Part model, mm, in its own coordinate system. A direction names the side the tool comes from. Round coordinates to 2 decimals unless told otherwise and drop trailing zeros. Write each loop counter-clockwise with the first axis right and the second up, starting at its lowest first coordinate (ties: lowest second). Pieces come first, ordered by that corner, then holes.
Solid Edge part; units mm, degrees
sketch "Sketch1" plane through (0, 0, 0) normal (0, 0, 1) x (1, 0, 0)
  circle A0 centre (0, 0) radius 12.5
  circle A1 centre (0, 0) radius 1.6
extrude "Protrusion1" add sketch "Sketch1" along normal blind 35
sketch "Sketch2" plane through (0, 0, 35) normal (0, 0, 1) x (1, 0, 0)
  circle A0 centre (0, 0) radius 12.5
  circle A1 centre (0, 0) radius 6
extrude "ExtrudedCutout_1" cut sketch "Sketch2" against normal blind 28
sketch "Sketch3" plane through (0, 0, 7) normal (0, 0, 1) x (1, 0, 0)
  circle A0 centre (0, 9.5) radius 1.6
extrude "Cutout1" cut sketch "Sketch3" against normal up to next
sketch "Sketch4" plane through (0, 0, 7) normal (0, 0, 1) x (1, 0, 0)
  circle A0 centre (0, 9.5) radius 3.25
extrude "ExtrudedCutout_3" cut sketch "Sketch4" against normal blind 3.5
pattern_circular "Pattern1" count 4 over 360 about axis through (0, 0, 7) along (0, 0, 1) of "Cutout1", "ExtrudedCutout_3"
hole "Hole_4" at (0, 0, 29) direction (0, 1, 0) diameter 2.013 end up to next
hole "Hole1" at (0, 0, 20) direction (0, 1, 0) diameter 2.013 end up to next
hole "Hole2" at (0, 0, 11) direction (0, 1, 0) diameter 2.013 end up to next
Q1. Cut at B-B on x = 10.5. Write the cut outline in (y, z).
Values follow:
outline: (-6.78, 0) - (-1.25, 0) - (-1.25, 3.5) - (-3.09, 3.5) - (-3.09, 7) - (-6.78, 7) - close; (1.25, 0) - (6.78, 0) - (6.78, 7) - (3.09, 7) - (3.09, 3.5) - (1.25, 3.5) - close
Q2. Cut at A-A on y = 4.5. Write the cut outline in (x, z).
Values follow:
outline: (-11.66, 0) - (11.66, 0) - (11.66, 7) - (3.97, 7) - (3.97, 35) - (-3.97, 35) - (-3.97, 7) - (-11.66, 7) - close; hole circle Ø2.01 at (0, 11); hole circle Ø2.01 at (0, 20); hole circle Ø2.01 at (0, 29)
Q3. Drop flat-ended pins along their axis: pin 1 (12 mm diameter, centred on y = -7, z = 7.5, fed in from +X); pin 2 (4 mm diameter, centred on x = -2.5, y = 10, fed in from +Z); pin 3 (5 mm diameter, centred on y = 2, z = 23, fed in from +X); pin 4 (2.5 mm diameter, centred on x = 9.5, y = 0, fed in from +Z). Give the stop position or say it passes through.
Values follow:
pin 1: stops at x = 12.42
pin 2: stops at z = 7
pin 3: stops at x = 6
pin 4: passes through
Q4. Cut at C-C on y = 9.5. Write the cut outline in (x, z).
Values follow:
outline: (-8.12, 0) - (-1.6, 0) - (-1.6, 3.5) - (-3.25, 3.5) - (-3.25, 7) - (-8.12, 7) - close; (1.6, 0) - (8.12, 0) - (8.12, 7) - (3.25, 7) - (3.25, 3.5) - (1.6, 3.5) - close
Q5. Which spindle directions (+Z, -Z, +X, -X, +Y, -Y) get a long thin tool onto all of the face, cutting with end or side? Do faces 1 (the flat face through (8, -1, 3.5)), 2 (the cylindrical face through (7.94, 0.35, 1.77)), 3 (the cylindrical face through (1, 3.6, 11.1)). Say none if no direction does.
Values follow:
face 1: +Z
face 2: +Z, -Z
face 3: +Y
Q6. Cut at D-D on x = 0. State how many separate pieces and enclosed holes the cut face has, plus the area to 3 significant figures.
Values follow:
separate pieces: 7
enclosed holes: 0
area: 306 mm2
Q7. Mould opens along Z. For faces 4 (the flat face through (0, -3, 0)), 5 (the flat face through (1.25, -1.25, 35)), 6 (the cylindrical face through (-0.122, 6.252, 5.274)), 7 (the cylindrical face through (1, 3.6, 20.1)) say: +Z half, -Z half, draft (parallel to the pull), parting line (faces both ways), or undercut.
Values follow:
face 4: -Z half
face 5: +Z half
face 6: draft
face 7: undercut
Q8. Wall check: L1, parallel to Z at x = 0, y = 2.45; L2, parallel to Y at x = 0, z = 1.65; L3, parallel to X at y = 2.25, z = 6. Give the ranges that are in metal, low to high.
Values follow:
L1: z = 0 to 9.99, 12.01 to 18.99, 21.01 to 27.99, 30.01 to 35
L2: y = -12.5 to -11.1, -7.9 to -1.6, 1.6 to 7.9, 11.1 to 12.5
L3: x = -12.3 to -11.85, -7.15 to 7.15, 11.85 to 12.3
